from build123d import *

# Parameters (mm, degrees)
SKETCH_1_R          = 42.5
EXTRUDE_1_DEPTH     = 3
SKETCH_2_R          = 4.15
CUT_EXTRUDE_1_DEPTH = 61.178899957
SKETCH_3_R          = 5.15
CUT_EXTRUDE_2_DEPTH = 61.178899957
EXTRUDE_START       = -1
SKETCH_4_R          = 4.15
SKETCH_4_R_2        = 3.15
EXTRUDE_1_2_DEPTH   = 1
CUT_EXTRUDE_3_REACH = 62.179
SKETCH_5_R          = 1.65
CUT_EXTRUDE_4_REACH = 62.179
SKETCH_7_R          = 2.15
CHAMFER_2_SIZE      = 0.4
EXTRUDE_START_2     = -3
EXTRUDE_3_DEPTH     = 3


with BuildPart() as part:
    # 草图1 → Extrude 1 (new body)
    with BuildSketch(Plane.XY):
        Circle(SKETCH_1_R)
    extrude(amount=-EXTRUDE_1_DEPTH)

    # 草图2 → 切除-拉伸1 (cut, through all)
    with BuildSketch(Plane.XY):
        with Locations((-32, 0)):
            Circle(SKETCH_2_R)
        with Locations((-16, 27.712812921)):
            Circle(SKETCH_2_R)
        with Locations((16, 27.712812921)):
            Circle(SKETCH_2_R)
        with Locations((32, 0)):
            Circle(SKETCH_2_R)
        with Locations((16, -27.712812921)):
            Circle(SKETCH_2_R)
        with Locations((-16, -27.712812921)):
            Circle(SKETCH_2_R)
    extrude(amount=-CUT_EXTRUDE_1_DEPTH, mode=Mode.SUBTRACT)

    # 草图3 → 切除-拉伸2 (cut, through all)
    with BuildSketch(Plane.XY):
        Circle(SKETCH_3_R)
    extrude(amount=-CUT_EXTRUDE_2_DEPTH, mode=Mode.SUBTRACT)

    # 草图4 → Extrude 1 2 (add)
    # profile 1 of 6: a face of its own
    with BuildSketch(Plane(origin=(0, 0, -3), x_dir=(-1, 0, 0), z_dir=(0, 0, -1)).offset(EXTRUDE_START)):
        with Locations((-16, 27.712812921)):
            Circle(SKETCH_4_R)
        with Locations((-16, 27.712812921)):
            Circle(SKETCH_4_R_2, mode=Mode.SUBTRACT)
    # profile 2 of 6: a face of its own
    with BuildSketch(Plane(origin=(0, 0, -3), x_dir=(-1, 0, 0), z_dir=(0, 0, -1)).offset(EXTRUDE_START)):
        with Locations((16, 27.712812921)):
            Circle(SKETCH_4_R)
        with Locations((16, 27.712812921)):
            Circle(SKETCH_4_R_2, mode=Mode.SUBTRACT)
    # profile 3 of 6: a face of its own
    with BuildSketch(Plane(origin=(0, 0, -3), x_dir=(-1, 0, 0), z_dir=(0, 0, -1)).offset(EXTRUDE_START)):
        with Locations((32, 0)):
            Circle(SKETCH_4_R)
        with Locations((32, 0)):
            Circle(SKETCH_4_R_2, mode=Mode.SUBTRACT)
    # profile 4 of 6: a face of its own
    with BuildSketch(Plane(origin=(0, 0, -3), x_dir=(-1, 0, 0), z_dir=(0, 0, -1)).offset(EXTRUDE_START)):
        with Locations((16, -27.712812921)):
            Circle(SKETCH_4_R)
        with Locations((16, -27.712812921)):
            Circle(SKETCH_4_R_2, mode=Mode.SUBTRACT)
    # profile 5 of 6: a face of its own
    with BuildSketch(Plane(origin=(0, 0, -3), x_dir=(-1, 0, 0), z_dir=(0, 0, -1)).offset(EXTRUDE_START)):
        with Locations((-16, -27.712812921)):
            Circle(SKETCH_4_R)
        with Locations((-16, -27.712812921)):
            Circle(SKETCH_4_R_2, mode=Mode.SUBTRACT)
    # profile 6 of 6: a face of its own
    with BuildSketch(Plane(origin=(0, 0, -3), x_dir=(-1, 0, 0), z_dir=(0, 0, -1)).offset(EXTRUDE_START)):
        with Locations((-32, 0)):
            Circle(SKETCH_4_R)
        with Locations((-32, 0)):
            Circle(SKETCH_4_R_2, mode=Mode.SUBTRACT)
    extrude(amount=EXTRUDE_1_2_DEPTH)

    # 草图5 → 切除-拉伸3 (cut, up to next)
    with BuildSketch(Plane(origin=(0, 0, -3), x_dir=(-1, 0, 0), z_dir=(0, 0, -1)), mode=Mode.PRIVATE) as cut_extrude_3_sk1:
        with Locations((-16.454482672, -9.5)):
            Circle(SKETCH_5_R)
    cut_extrude_3_tool1 = extrude(cut_extrude_3_sk1.sketch, amount=-CUT_EXTRUDE_3_REACH, mode=Mode.PRIVATE) & part.part
    # 草图5 → 切除-拉伸3 (cut, up to next)
    with BuildSketch(Plane(origin=(0, 0, -3), x_dir=(-1, 0, 0), z_dir=(0, 0, -1)), mode=Mode.PRIVATE) as cut_extrude_3_sk2:
        with Locations((0, 19)):
            Circle(SKETCH_5_R)
    cut_extrude_3_tool2 = extrude(cut_extrude_3_sk2.sketch, amount=-CUT_EXTRUDE_3_REACH, mode=Mode.PRIVATE) & part.part
    # 草图5 → 切除-拉伸3 (cut, up to next)
    with BuildSketch(Plane(origin=(0, 0, -3), x_dir=(-1, 0, 0), z_dir=(0, 0, -1)), mode=Mode.PRIVATE) as cut_extrude_3_sk3:
        with Locations((16.454482672, -9.5)):
            Circle(SKETCH_5_R)
    cut_extrude_3_tool3 = extrude(cut_extrude_3_sk3.sketch, amount=-CUT_EXTRUDE_3_REACH, mode=Mode.PRIVATE) & part.part
    add(cut_extrude_3_tool1.solids().sort_by_distance((16.454483, -9.5, -3))[0], mode=Mode.SUBTRACT)
    add(cut_extrude_3_tool2.solids().sort_by_distance((0, 19, -3))[0], mode=Mode.SUBTRACT)
    add(cut_extrude_3_tool3.solids().sort_by_distance((-16.454483, -9.5, -3))[0], mode=Mode.SUBTRACT)

    # 草图7 → 切除-拉伸4 (cut, up to next)
    with BuildSketch(Plane.XY, mode=Mode.PRIVATE) as cut_extrude_4_sk1:
        with Locations((9.526279442, 5.5)):
            Circle(SKETCH_7_R)
    cut_extrude_4_tool1 = extrude(cut_extrude_4_sk1.sketch, amount=-CUT_EXTRUDE_4_REACH, mode=Mode.PRIVATE) & part.part
    # 草图7 → 切除-拉伸4 (cut, up to next)
    with BuildSketch(Plane.XY, mode=Mode.PRIVATE) as cut_extrude_4_sk2:
        with Locations((0, -11)):
            Circle(SKETCH_7_R)
    cut_extrude_4_tool2 = extrude(cut_extrude_4_sk2.sketch, amount=-CUT_EXTRUDE_4_REACH, mode=Mode.PRIVATE) & part.part
    # 草图7 → 切除-拉伸4 (cut, up to next)
    with BuildSketch(Plane.XY, mode=Mode.PRIVATE) as cut_extrude_4_sk3:
        with Locations((-9.526279442, 5.5)):
            Circle(SKETCH_7_R)
    cut_extrude_4_tool3 = extrude(cut_extrude_4_sk3.sketch, amount=-CUT_EXTRUDE_4_REACH, mode=Mode.PRIVATE) & part.part
    add(cut_extrude_4_tool1.solids().sort_by_distance((9.526279, 5.5, 0))[0], mode=Mode.SUBTRACT)
    add(cut_extrude_4_tool2.solids().sort_by_distance((0, -11, 0))[0], mode=Mode.SUBTRACT)
    add(cut_extrude_4_tool3.solids().sort_by_distance((-9.526279, 5.5, 0))[0], mode=Mode.SUBTRACT)

    # 倒角2
    chamfer_2_edges = [part.edges().sort_by_distance(p)[0] for p in [
        (-36.15, 0, 0),
        (-20.15, -27.712812921, 0),
        (11.85, -27.712812921, 0),
        (27.85, 0, 0),
        (11.85, 27.712812921, 0),
        (-20.15, 27.712812921, 0),
        (-5.15, 0, 0),
        (18.104482672, -9.5, 0),
        (1.65, 19, 0),
        (-14.804482672, -9.5, 0),
    ]]
    chamfer(chamfer_2_edges, length=CHAMFER_2_SIZE)

    # 草图8 → 拉伸-薄壁3 (add)
    with BuildSketch(Plane.XY.offset(EXTRUDE_START_2)):
        Polygon((33.056079661, 27.745190528), (40.556079661, 14.754809472), (39.690054257, 14.254809472), (32.190054257, 27.245190528), align=None)
    extrude(amount=EXTRUDE_3_DEPTH)


solid = part.part
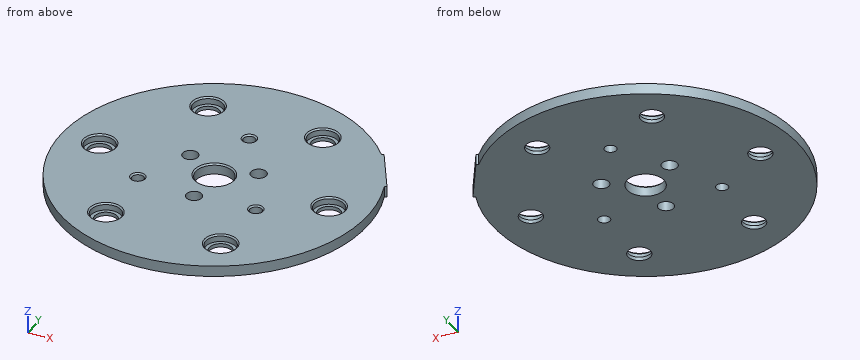
Model file for the job. Use its own axes, mm. Coordinates: 2 decimals unless noted, no trailing zeros. Loops run counter-clockwise (first coordinate to the right, second up) from the corner with the lowest first, then second, coordinate; pieces in that order, holes last. Notation, with made-up numbers: (-32, 10) -> (14, 10) arc R15 cw to (14, 22) -> close; hole circle Ø6 at (62.5, -3). An arc over 180 degrees is marked (long way). Use one line per item in the form item = value. Start each with the question number.
(1) Cut at A-A on y = 0. Give the number of separate pieces and of enclosed holes in the cut face, and give its area (3 significant figures).
(2) Flat gauge pins, fed straight in: pin 1 (2 mm diameter, centred on x = -16.45, y = -9.5, fed in from -Z); pin 2 (7 mm diameter, centred on x = 16, y = -27.71, fed in from +Z); pin 3 (1.5 mm diameter, centred on x = 15.5, z = -1.5, fed in from +Y). Where does each tip first touch, or does it go through?
(3) Cut at D-D on x = -24.5. Give the cut face in (y, z).
(4) Probe probe 1 along Y at (x, z) = (-19, -1.3); probe 2 along Y at (x, z) = (15, -0.8); probe 3 along Y at (x, z) = (16, -1.4). List the from-to ranges inside material, lowest first. Write a range as from..to.
(5) Cut at B-B on y = 19. Give the cut face in (x, z).
Values:
q1.separate_pieces = 4
q1.enclosed_holes = 0
q1.area = 178 mm2
q2.pin_1 = through
q2.pin_2 = -2
q2.pin_3 = 39.86
q3.outline = (-34.73, -3) -> (34.73, -3) -> (34.73, 0) -> (-34.73, 0) -> close
q4.probe_1 = -38.02..-30.58, -24.85..24.85, 30.58..38.02
q4.probe_2 = -39.76..-31.74, -23.69..-10.28, -8.72..23.69, 31.74..39.76
q4.probe_3 = -39.37..-31.86, -23.56..-11.09, -7.91..23.56, 31.86..39.37
q5.outline = (-38.02, -3) -> (-1.65, -3) -> (-1.65, -0.4) -> (-2.05, 0) -> (-38.02, 0) -> close; (1.65, -3) -> (38.11, -3) -> (38.11, 0) -> (2.05, 0) -> (1.65, -0.4) -> close
